Could you check a few things on this model? Use its own coordinates, in mm. A direction names the side the tool comes from. Coordinates: 2 decimals unless noted, no trailing zeros. Write each loop counter-clockwise with the first axis right and the second up, starting at its lowest first coordinate (ties: lowest second). Pieces come first, ordered by that corner, then holes. Notation, with made-up numbers: (56.5, -1) - (70.5, -1) arc R25 cw to (70.5, 23) - close; hole circle Ø3 at (-5.75, 3). An arc over 180 degrees is marked (long way). Answer as a JSON object with one key per item and string values. Group by question number.
1) On a 3-axis mill with a long thin cutter (end or side, diameter ignored), from which of +Z, -Z, +X, -X, +Y, -Y can I reach the whole of each face in a straight line? I mean faces 1 (the flat face through (4, 5, -14.75)), 2 (the flat face through (0.7, 7, -17)), 3 (the flat face through (6, 12, 5.2)), 4 (the flat face through (2.3, 7, 17)), 5 (the flat face through (1.2, 12.5, -9)). Say none if no direction works.
2) Will these pins go through, and if not, where does the flat tip stop? pin 1 Ø1.5 at (y, z) = (8.5, 18) entering from -X; pin 2 Ø1.5 at (x, z) = (1, 1.5) entering from +Y; pin 3 Ø3.5 at (x, y) = (5, 5) entering from +Z.
3) Please list where these lines run through material, in increasing order: line 1 along Z through (x, y) = (7.25, 3); line 2 along Z through (x, y) = (7.5, 9.5); line 3 along Y through (x, z) = (1, 5).
4) We'd pull the mould along Z, two halves only. Please class faces 6 (the flat face through (2, 10.8, 0)), 7 (the flat face through (2, 7, 18.8)), 8 (the flat face through (3.1, 0, -15.6)): released by +Z, released by -Z, zero draft, split by the parting line, or undercut.
5) If we section it at C-C (z = -12.5): Write out the boundary of the cut face in (x, y).
6) If we section it at A-A (y = 7.5): Write out the boundary of the cut face in (x, z), plus the area to 3 significant figures.
7) If we section it at B-B (x = 6.5): Write out the boundary of the cut face in (y, z), plus the area to 3 significant figures.
8) If we section it at D-D (y = 9.5): Write out the boundary of the cut face in (x, z), plus the area to 3 significant figures.
```python
from build123d import *

# Parameters (mm, degrees)
SKETCH1_W           = 38
SKETCH1_H           = 13
BOSS_EXTRUDE1_DEPTH = 3
CUT_EXTRUDE1_DEPTH  = 24.216373532
SKETCH3_W           = 29.5
SKETCH3_H           = 10.8
CUT_EXTRUDE2_DEPTH  = 3
BOSS_EXTRUDE2_DEPTH = 5.85
SKETCH5_W           = 9.75
SKETCH5_H           = 2.4
BOSS_EXTRUDE3_DEPTH = 1.5
CUT_EXTRUDE3_DEPTH  = 10
SKETCH7_W           = 18
SKETCH7_H           = 1
CUT_EXTRUDE4_DEPTH  = 2.4


with BuildPart() as part:
    # Sketch1 → Boss-Extrude1 (new body)
    with BuildSketch(Plane(origin=(0, 0, 0), x_dir=(0, 0, -1), z_dir=(1, 0, 0))):
        with Locations((0, 6.5)):
            Rectangle(SKETCH1_W, SKETCH1_H)
    extrude(amount=BOSS_EXTRUDE1_DEPTH)

    # Sketch2 → Cut-Extrude1 (cut, through all)
    with BuildSketch(Plane(origin=(0, 13, 0), x_dir=(1, 0, 0), z_dir=(0, 1, 0))):
        Polygon((0.7, -18.8), (0.7, -15.8), (0, -15.8), (0, -19), (3, -19), (3, -15.8), (2.3, -15.8), (2.3, -18.8), align=None)
        Polygon((2.3, 18.8), (2.3, 15.8), (3, 15.8), (3, 19), (0, 19), (0, 15.8), (0.7, 15.8), (0.7, 18.8), align=None)
    extrude(amount=-CUT_EXTRUDE1_DEPTH, mode=Mode.SUBTRACT)

    # Sketch3 → Cut-Extrude2 (cut)
    with BuildSketch(Plane(origin=(3, 0, 0), x_dir=(0, 0, -1), z_dir=(1, 0, 0))):
        with Locations((0, 5.4)):
            Rectangle(SKETCH3_W, SKETCH3_H)
    extrude(amount=-CUT_EXTRUDE2_DEPTH, mode=Mode.SUBTRACT)

    # Sketch4 → Boss-Extrude2 (add)
    with BuildSketch(Plane(origin=(3, 0, 0), x_dir=(0, 0, -1), z_dir=(1, 0, 0))):
        Polygon((-15.8, 13), (-15.8, 0), (-14.75, 0), (-14.75, 10.8), (14.75, 10.8), (14.75, 0), (15.8, 0), (15.8, 13), align=None)
    extrude(amount=BOSS_EXTRUDE2_DEPTH)

    # Sketch5 → Boss-Extrude3 (add)
    with BuildSketch(Plane(origin=(8.85, 0, 0), x_dir=(0, 0, -1), z_dir=(1, 0, 0))):
        with Locations((-9.875, 9.6)):
            Rectangle(SKETCH5_W, SKETCH5_H)
        with Locations((9.875, 9.6)):
            Rectangle(SKETCH5_W, SKETCH5_H)
    extrude(amount=-BOSS_EXTRUDE3_DEPTH)

    # Sketch6 → Cut-Extrude3 (cut)
    with BuildSketch(Plane(origin=(0, 13, 0), x_dir=(1, 0, 0), z_dir=(0, 1, 0))):
        Polygon((8.85, 5.2), (2.35, 5.2), (2.35, 0), (2.35, -5.2), (8.85, -5.2), align=None)
    extrude(amount=-CUT_EXTRUDE3_DEPTH, mode=Mode.SUBTRACT)

    # Sketch7 → Cut-Extrude4 (cut)
    with BuildSketch(Plane.ZY):
        with Locations((0, 12.5)):
            Rectangle(SKETCH7_W, SKETCH7_H)
    extrude(amount=-CUT_EXTRUDE4_DEPTH, mode=Mode.SUBTRACT)


solid = part.part
```
Here are the results:
{
 "1": {"face 1": "-X, -Y", "face 2": "-Z, -X, +Y, -Y", "face 3": "+X, +Y, -Y", "face 4": "+Z, +X, +Y, -Y", "face 5": "-X, +Y"},
 "2": {"pin 1": "stops at x = 0.7", "pin 2": "stops at y = 12", "pin 3": "stops at z = 15.8"},
 "3": {"line 1": "z = -15.8 to -14.75, 14.75 to 15.8", "line 2": "z = -15.8 to -5.2, 5.2 to 15.8", "line 3": "y = 10.8 to 12"},
 "4": {"face 6": "undercut", "face 7": "released by +Z", "face 8": "zero draft"},
 "5": {"outline": "(0, 10.8) - (7.35, 10.8) - (7.35, 8.4) - (8.85, 8.4) - (8.85, 13) - (0, 13) - close"},
 "6": {"outline": "(0, -15.8) - (0.7, -15.8) - (0.7, -18.8) - (2.3, -18.8) - (2.3, -15.8) - (8.85, -15.8) - (8.85, -14.75) - (0, -14.75) - close; (0, 14.75) - (8.85, 14.75) - (8.85, 15.8) - (2.3, 15.8) - (2.3, 18.8) - (0.7, 18.8) - (0.7, 15.8) - (0, 15.8) - close", "area": "28.2 mm²"},
 "7": {"outline": "(0, -15.8) - (13, -15.8) - (13, -5.2) - (10.8, -5.2) - (10.8, -14.75) - (0, -14.75) - close; (0, 14.75) - (10.8, 14.75) - (10.8, 5.2) - (13, 5.2) - (13, 15.8) - (0, 15.8) - close", "area": "69.3 mm²"},
 "8": {"outline": "(0, -15.8) - (0.7, -15.8) - (0.7, -18.8) - (2.3, -18.8) - (2.3, -15.8) - (8.85, -15.8) - (8.85, -5.2) - (7.35, -5.2) - (7.35, -14.75) - (0, -14.75) - close; (0, 14.75) - (7.35, 14.75) - (7.35, 5.2) - (8.85, 5.2) - (8.85, 15.8) - (2.3, 15.8) - (2.3, 18.8) - (0.7, 18.8) - (0.7, 15.8) - (0, 15.8) - close", "area": "56.8 mm²"}
}
